Input: part model. Units: mm. Frame: model coordinates. A direction names the side the tool comes from. Coordinates: 2 decimals unless noted, no trailing zeros. Loops run counter-clockwise (first coordinate to the right, second up) from the corner with the lowest first, then second, coordinate; pieces in that order, holes last.
```python
from build123d import *

# Parameters (mm, degrees)
SKETCH1_W                      = 46.48
SKETCH1_H                      = 30.48
SKETCH1_R                      = 3.175
BOSS_EXTRUDE1_DEPTH            = 9.46
SKETCH2_W                      = 46.48
SKETCH2_H                      = 5.24
BOSS_EXTRUDE2_DEPTH            = 53
CUT_EXTRUDE1_REACH             = 70.364
SKETCH4_R                      = 3.96875
CUT_EXTRUDE1_DIRECTION_2_REACH = 70.364
CUT_EXTRUDE3_REACH             = 70.364
CUT_EXTRUDE3_DIRECTION_2_REACH = 70.364
CUT_EXTRUDE4_DEPTH             = 9.46
BOSS_EXTRUDE3_DEPTH            = 9.46
FILLET3_R                      = 6.35
CUT_EXTRUDE5_DEPTH             = 2.54


with BuildPart() as part:
    # Sketch1 → Boss-Extrude1 (new body)
    with BuildSketch(Plane.XY):
        Rectangle(SKETCH1_W, SKETCH1_H)
        with Locations((15.24, 0)):
            Circle(SKETCH1_R, mode=Mode.SUBTRACT)
        with Locations((-15.24, 0)):
            Circle(SKETCH1_R, mode=Mode.SUBTRACT)
    extrude(amount=BOSS_EXTRUDE1_DEPTH)

    # Sketch2 → Boss-Extrude2 (add)
    with BuildSketch(Plane.XY.offset(9.46)):
        with Locations((0, 12.62)):
            Rectangle(SKETCH2_W, SKETCH2_H)
        with Locations((0, -12.62)):
            Rectangle(SKETCH2_W, SKETCH2_H)
    extrude(amount=BOSS_EXTRUDE2_DEPTH)

    # Cut-Extrude1: up to this face of the body (flat: up to its plane)
    cut_extrude1_end = Plane(part.part.faces().sort_by_distance((0, -15.24, 31.23))[0])
    # Sketch4 → Cut-Extrude1 (cut, up to the picked face)
    with BuildSketch(Plane(origin=(0, 0, 0), x_dir=(1, 0, 0), z_dir=(0, 1, 0)), mode=Mode.PRIVATE) as cut_extrude1_sk1:
        with Locations(Location((0, -25.8481308, 0), (0, 0, 270))):
            Circle(SKETCH4_R)
    cut_extrude1_tool1 = split(extrude(cut_extrude1_sk1.sketch, amount=-CUT_EXTRUDE1_REACH, mode=Mode.PRIVATE), bisect_by=cut_extrude1_end, keep=Keep.BOTH, mode=Mode.PRIVATE)
    add(cut_extrude1_tool1.solids().sort_by(Axis((0, 0, 25.848131), (0, -1, 0)))[0], mode=Mode.SUBTRACT)

    # Cut-Extrude1 direction 2: up to this face of the body (flat: up to its plane)
    cut_extrude1_direction_2_end = Plane(part.part.faces().sort_by_distance((0, 15.24, 31.23))[0])
    # Sketch4 → Cut-Extrude1 direction 2 (cut, up to the picked face)
    with BuildSketch(Plane(origin=(0, 0, 0), x_dir=(1, 0, 0), z_dir=(0, 1, 0)), mode=Mode.PRIVATE) as cut_extrude1_direction_2_sk1:
        with Locations(Location((0, -25.8481308, 0), (0, 0, 270))):
            Circle(SKETCH4_R)
    cut_extrude1_direction_2_tool1 = split(extrude(cut_extrude1_direction_2_sk1.sketch, amount=CUT_EXTRUDE1_DIRECTION_2_REACH, mode=Mode.PRIVATE), bisect_by=cut_extrude1_direction_2_end, keep=Keep.BOTH, mode=Mode.PRIVATE)
    add(cut_extrude1_direction_2_tool1.solids().sort_by(Axis((0, 0, 25.848131), (0, 1, 0)))[0], mode=Mode.SUBTRACT)

    # Cut-Extrude3: up to this face of the body (flat: up to its plane)
    cut_extrude3_end = Plane(part.part.faces().sort_by_distance((0, -15.24, 31.323322986))[0])
    # Sketch6 → Cut-Extrude3 (cut, up to the picked face)
    with BuildSketch(Plane(origin=(0, 0, 0), x_dir=(1, 0, 0), z_dir=(0, 1, 0)), mode=Mode.PRIVATE) as cut_extrude3_sk1:
        with BuildLine():
            Line((-8.4418692, -25.8481308), (-8.4418692, -17.46))
            Line((-8.4418692, -17.46), (-8.4418692, -9.46))
            Line((-8.4418692, -9.46), (-16.4418692, -9.46))
            Line((-16.4418692, -9.46), (-23.24, -9.46))
            Line((-23.24, -9.46), (-23.24, -62.46))
            Line((-23.24, -62.46), (23.24, -62.46))
            Line((23.24, -62.46), (23.24, -9.46))
            Line((23.24, -9.46), (16.4418692, -9.46))
            Line((16.4418692, -9.46), (8.4418692, -9.46))
            Line((8.4418692, -9.46), (8.4418692, -17.46))
            Line((8.4418692, -17.46), (8.4418692, -25.8481308))
            ThreePointArc((8.4418692, -25.8481308), (0, -34.29), (-8.4418692, -25.8481308))
        make_face()
    cut_extrude3_tool1 = split(extrude(cut_extrude3_sk1.sketch, amount=-CUT_EXTRUDE3_REACH, mode=Mode.PRIVATE), bisect_by=cut_extrude3_end, keep=Keep.BOTH, mode=Mode.PRIVATE)
    add(cut_extrude3_tool1.solids().sort_by(Axis((0, 0, 38.753518), (0, -1, 0)))[0], mode=Mode.SUBTRACT)

    # Cut-Extrude3 direction 2: up to this face of the body (flat: up to its plane)
    cut_extrude3_direction_2_end = Plane(part.part.faces().sort_by_distance((0, 15.24, 31.323322986))[0])
    # Sketch6 → Cut-Extrude3 direction 2 (cut, up to the picked face)
    with BuildSketch(Plane(origin=(0, 0, 0), x_dir=(1, 0, 0), z_dir=(0, 1, 0)), mode=Mode.PRIVATE) as cut_extrude3_direction_2_sk1:
        with BuildLine():
            Line((-8.4418692, -25.8481308), (-8.4418692, -17.46))
            Line((-8.4418692, -17.46), (-8.4418692, -9.46))
            Line((-8.4418692, -9.46), (-16.4418692, -9.46))
            Line((-16.4418692, -9.46), (-23.24, -9.46))
            Line((-23.24, -9.46), (-23.24, -62.46))
            Line((-23.24, -62.46), (23.24, -62.46))
            Line((23.24, -62.46), (23.24, -9.46))
            Line((23.24, -9.46), (16.4418692, -9.46))
            Line((16.4418692, -9.46), (8.4418692, -9.46))
            Line((8.4418692, -9.46), (8.4418692, -17.46))
            Line((8.4418692, -17.46), (8.4418692, -25.8481308))
            ThreePointArc((8.4418692, -25.8481308), (0, -34.29), (-8.4418692, -25.8481308))
        make_face()
    cut_extrude3_direction_2_tool1 = split(extrude(cut_extrude3_direction_2_sk1.sketch, amount=CUT_EXTRUDE3_DIRECTION_2_REACH, mode=Mode.PRIVATE), bisect_by=cut_extrude3_direction_2_end, keep=Keep.BOTH, mode=Mode.PRIVATE)
    add(cut_extrude3_direction_2_tool1.solids().sort_by(Axis((0, 0, 38.753518), (0, 1, 0)))[0], mode=Mode.SUBTRACT)

    # Sketch7 → Cut-Extrude4 (cut)
    with BuildSketch(Plane.XY):
        with BuildLine():
            ThreePointArc((-15.24, -7), (-22.24, 0), (-15.24, 7))
            Line((-15.24, 7), (-8.4418692, 7))
            Line((-8.4418692, 7), (-8.4418692, 15.24))
            Line((-8.4418692, 15.24), (-23.24, 15.24))
            Line((-23.24, 15.24), (-23.24, -15.24))
            Line((-23.24, -15.24), (-8.4418692, -15.24))
            Line((-8.4418692, -15.24), (-8.4418692, -7))
            Line((-8.4418692, -7), (-15.24, -7))
        make_face()
        with BuildLine():
            Line((8.4418692, 15.24), (8.4418692, 7))
            Line((8.4418692, 7), (15.24, 7))
            ThreePointArc((15.24, 7), (22.24, 0), (15.24, -7))
            Line((15.24, -7), (8.4418692, -7))
            Line((8.4418692, -7), (8.4418692, -15.24))
            Line((8.4418692, -15.24), (23.24, -15.24))
            Line((23.24, -15.24), (23.24, 15.24))
            Line((23.24, 15.24), (8.4418692, 15.24))
        make_face()
    extrude(amount=CUT_EXTRUDE4_DEPTH, mode=Mode.SUBTRACT)

    # Sketch8 → Boss-Extrude3 (add)
    with BuildSketch(Plane.XY):
        with BuildLine():
            Line((8.4418692, -15.24), (19.846982329, -5.27026696))
            ThreePointArc((19.846982329, -5.27026696), (17.700501096, -6.553314761), (15.24, -7))
            Line((15.24, -7), (8.4418692, -7))
            Line((8.4418692, -7), (8.4418692, -15.24))
        make_face()
        with BuildLine():
            ThreePointArc((-19.846982329, -5.27026696), (-17.700501096, -6.553314761), (-15.24, -7))
            Line((-15.24, -7), (-8.4418692, -7))
            Line((-8.4418692, -7), (-8.4418692, -15.24))
            Line((-8.4418692, -15.24), (-19.846982329, -5.27026696))
        make_face()
        with BuildLine():
            Line((8.4418692, 15.24), (19.846982329, 5.27026696))
            ThreePointArc((19.846982329, 5.27026696), (17.700501096, 6.553314761), (15.24, 7))
            Line((15.24, 7), (8.4418692, 7))
            Line((8.4418692, 7), (8.4418692, 15.24))
        make_face()
        with BuildLine():
            Line((-8.4418692, 15.24), (-19.846982329, 5.27026696))
            ThreePointArc((-19.846982329, 5.27026696), (-17.700501096, 6.553314761), (-15.24, 7))
            Line((-15.24, 7), (-8.4418692, 7))
            Line((-8.4418692, 7), (-8.4418692, 15.24))
        make_face()
    extrude(amount=BOSS_EXTRUDE3_DEPTH)

    # Fillet3
    # the kernel refuses this fillet: 6.35 mm, written as the material it adds along each edge
    with BuildSketch(Plane(origin=(8.4418692, -10, 9.46), x_dir=(0, 0, 1), z_dir=(0, -1, 0))) as fillet3_piece_1_section:
        with BuildLine():
            CenterArc((FILLET3_R, -FILLET3_R), FILLET3_R, 90, 90)
            Line((0, -FILLET3_R), (0, 0))
            Line((0, 0), (FILLET3_R, 0))
        make_face()
    fillet3_piece_1 = extrude(amount=5.24, mode=Mode.PRIVATE)
    fillet3_piece_1 = split(fillet3_piece_1, bisect_by=Plane(origin=(10.547300474, -13.399545855, 11.138669317), z_dir=(-0.6581403326503757, 0.7528952799286586, 0)), keep=Keep.TOP, mode=Mode.PRIVATE)
    add(fillet3_piece_1)
    with BuildSketch(Plane(origin=(-8.4418692, -10, 9.46), x_dir=(0, 0, 1), z_dir=(0, -1, 0))) as fillet3_piece_2_section:
        with BuildLine():
            CenterArc((FILLET3_R, FILLET3_R), FILLET3_R, 180, 90)
            Line((0, FILLET3_R), (0, 0))
            Line((0, 0), (FILLET3_R, 0))
        make_face()
    fillet3_piece_2 = extrude(amount=5.24, mode=Mode.PRIVATE)
    fillet3_piece_2 = split(fillet3_piece_2, bisect_by=Plane(origin=(-10.547300474, -13.399545855, 11.138669317), z_dir=(0.6581403326503753, 0.7528952799286588, 0)), keep=Keep.TOP, mode=Mode.PRIVATE)
    add(fillet3_piece_2)
    with BuildSketch(Plane(origin=(8.4418692, 10, 9.46), x_dir=(1, 0, 0), z_dir=(0, 1, 0))) as fillet3_piece_3_section:
        with BuildLine():
            CenterArc((FILLET3_R, -FILLET3_R), FILLET3_R, 90, 90)
            Line((0, -FILLET3_R), (0, 0))
            Line((0, 0), (FILLET3_R, 0))
        make_face()
    fillet3_piece_3 = extrude(amount=5.24, mode=Mode.PRIVATE)
    fillet3_piece_3 = split(fillet3_piece_3, bisect_by=Plane(origin=(10.547300473, 13.399545855, 11.138669317), z_dir=(-0.6581403326503754, -0.7528952799286586, 0)), keep=Keep.TOP, mode=Mode.PRIVATE)
    add(fillet3_piece_3)
    with BuildSketch(Plane(origin=(-8.4418692, 10, 9.46), x_dir=(-1, 0, 0), z_dir=(0, 1, 0))) as fillet3_piece_4_section:
        with BuildLine():
            CenterArc((FILLET3_R, FILLET3_R), FILLET3_R, 180, 90)
            Line((0, FILLET3_R), (0, 0))
            Line((0, 0), (FILLET3_R, 0))
        make_face()
    fillet3_piece_4 = extrude(amount=5.24, mode=Mode.PRIVATE)
    fillet3_piece_4 = split(fillet3_piece_4, bisect_by=Plane(origin=(-10.547300473, 13.399545855, 11.138669317), z_dir=(0.6581403326503757, -0.7528952799286586, 0)), keep=Keep.TOP, mode=Mode.PRIVATE)
    add(fillet3_piece_4)

    # Sketch10 → Cut-Extrude5 (cut)
    with BuildSketch(Plane.XY):
        with BuildLine():
            Line((-8.4418692, 15.24), (-19.846982329, 5.27026696))
            ThreePointArc((-19.846982329, 5.27026696), (-22.24, 0), (-19.846982329, -5.27026696))
            Line((-19.846982329, -5.27026696), (-8.4418692, -15.24))
            Line((-8.4418692, -15.24), (8.4418692, -15.24))
            Line((8.4418692, -15.24), (19.846982329, -5.27026696))
            ThreePointArc((19.846982329, -5.27026696), (22.24, 0), (19.846982329, 5.27026696))
            Line((19.846982329, 5.27026696), (8.4418692, 15.24))
            Line((8.4418692, 15.24), (-8.4418692, 15.24))
        make_face()
    extrude(amount=CUT_EXTRUDE5_DEPTH, mode=Mode.SUBTRACT)


solid = part.part
```
Item 1: Line query: L1, parallel to Z at x = 0, y = 12.8; L2, parallel to X at y = 0, z = 6.25 (3 decimals); L3, parallel to Y at x = -2.5, z = 11. Output: solid intervals per line, ascending.
Result:
L1: z = 2.54 to 21.88, 29.82 to 34.29
L2: x = -22.24 to -18.415, -12.065 to 12.065, 18.415 to 22.24
L3: y = -15.24 to -10, 10 to 15.24
Item 2: Section query A-A (x = 0). Output: boundary loops of the cut face in (y, z).
Result:
outline: (-15.24, 2.54) - (15.24, 2.54) - (15.24, 21.88) - (10, 21.88) - (10, 9.46) - (-10, 9.46) - (-10, 21.88) - (-15.24, 21.88) - close; (-15.24, 29.82) - (-10, 29.82) - (-10, 34.29) - (-15.24, 34.29) - close; (10, 29.82) - (15.24, 29.82) - (15.24, 34.29) - (10, 34.29) - close
Item 3: Section query C-C (x = -15.24). Output: boundary loops of the cut face in (y, z) (3 decimals), then the cut area to 3 significant figures.
Result:
outline: (-9.297, 2.54) - (-3.175, 2.54) - (-3.175, 9.46) - (-9.297, 9.46) - close; (3.175, 2.54) - (9.297, 2.54) - (9.297, 9.46) - (3.175, 9.46) - close
area: 84.7 mm2
Item 4: Section query B-B (z = 27.5). Output: boundary loops of the cut face in (x, y).
Result:
outline: (-8.28, -15.24) - (-3.61, -15.24) - (-3.61, -10) - (-8.28, -10) - close; (-8.28, 10) - (-3.61, 10) - (-3.61, 15.24) - (-8.28, 15.24) - close; (3.61, -15.24) - (8.28, -15.24) - (8.28, -10) - (3.61, -10) - close; (3.61, 10) - (8.28, 10) - (8.28, 15.24) - (3.61, 15.24) - close
Item 5: Contact query for flat-ended pins moving along their axis: P1, Ø7.5, axis at x = 15.24, y = 0, coming from the +Z side; P2, Ø2.5, axis at y = 12.5, z = 23, coming from the -X side; P3, Ø4, axis at y = -11.5, z = 19, coming from the +X side. Output: stop coordinate, or through.
Result:
P1: stops at z = 9.46
P2: stops at x = -8.44
P3: stops at x = 8.44
Item 6: Reachability of faces 5 (the face through (0, 15.24, 15)), 6 (the face through (0, 0, 9.46)), 7 (the face through (8.442, 13, 21)) from +Z, -Z, +X, -X, +Y, -Y: full face, straight path, thin tool, end or side. Return the list, or none.
Result:
face 5: +Z, -Z, +X, -X, +Y
face 6: +Z, +X, -X
face 7: +Z, +X, +Y, -Y
Item 7: Section query D-D (z = 6.5). Output: boundary loops of the cut face in (x, y) (3 decimals).
Result:
outline: (-19.847, -5.27) - (-8.442, -15.24) - (8.442, -15.24) - (19.847, -5.27) arc R7 ccw to (19.847, 5.27) - (8.442, 15.24) - (-8.442, 15.24) - (-19.847, 5.27) arc R7 ccw to start; hole circle Ø6.35 at (-15.24, 0); hole circle Ø6.35 at (15.24, 0)
Item 8: Mould query, pull axis Y, two halves, no side actions, for faces 1 (the face through (0, -10, 19)), 2 (the face through (-17.58, 2.146, 5.952)), 3 (the face through (-8.442, 13, 21)), 4 (the face through (22.24, 0.08, 5.95)). Classes: +Y half, -Y half, draft (parallel to the pull), parting line (faces both ways), or undercut.
Result:
face 1: undercut
face 2: undercut
face 3: draft
face 4: parting line
